from build123d import *

# Parameters (mm, degrees)
SKETCH1_R           = 9.2
BOSS_EXTRUDE1_DEPTH = 65
SKETCH2_W           = 10
SKETCH2_H           = 12.398416249
CUT_EXTRUDE3_DEPTH  = 68.723466712


with BuildPart() as part:
    # Sketch1 → Boss-Extrude1 (new body)
    with BuildSketch(Plane.XY):
        with BuildLine():
            Line((-7, -9.746794345), (-7, -14.746794345))
            Line((-7, -14.746794345), (7, -14.746794345))
            Line((7, -14.746794345), (7, -9.746794345))
            ThreePointArc((7, -9.746794345), (0, 12), (-7, -9.746794345))
        make_face()
        Circle(SKETCH1_R, mode=Mode.SUBTRACT)
    extrude(amount=BOSS_EXTRUDE1_DEPTH)

    # Sketch2 → Cut-Extrude3 (cut, through all)
    with BuildSketch(Plane.XY):
        with Locations((0, -6.800791875)):
            Rectangle(SKETCH2_W, SKETCH2_H)
    extrude(amount=CUT_EXTRUDE3_DEPTH, mode=Mode.SUBTRACT)


solid = part.part
Part model, mm, in its own coordinate system. A direction names the side the tool comes from. Coordinates: 2 decimals unless noted, no trailing zeros. Loops run counter-clockwise (first coordinate to the right, second up) from the corner with the lowest first, then second, coordinate; pieces in that order, holes last. Notation, with made-up numbers: (75.25, 2) -> (89.25, 2) arc R18 cw to (89.25, 23) -> close; hole circle Ø1 at (-40, 11.25). An arc over 180 degrees is marked (long way). Use a Markdown table: item, result. Add a question column.
Item 1: Which spindle directions (+Z, -Z, +X, -X, +Y, -Y) get a long thin tool onto all of the face, cutting with end or side? Do faces 4 (the flat face through (9, 3, 0)), 5 (the flat face through (-7, -12, 32)), 6 (the flat face through (5, -10, 32)). Say none if no direction does.
Item 2: Pull direction X, two halves, no side cores. Call faces 1 (the flat face through (7, -12, 32)), 2 (the flat face through (-5, -10, 32)), 3 (the flat face through (9, 3, 65)): +X half, -X half, draft (parallel to the pull), parting line (faces both ways), or undercut.
Item 3: Flat gauge pins, fed straight in: P1, Ø3, axis at y = 7, z = 55.5, coming from the -X side; P2, Ø1.5, axis at y = -12, z = 47.5, coming from the +X side; P3, Ø3, axis at x = 8.5, z = 47, coming from the +Y side; P4, Ø11, axis at x = 0, y = 0, coming from the -Z side. Where does each tip first touch, or does it go through?
Item 4: Band-saw the part on A-A on y = 0. Write the cut outline in (x, z), plus the area to 3 significant figures.
Item 5: Band-saw the part on B-B on x = 0. Write the cut outline in (y, z), plus the area to 3 significant figures.
Item 6: Probe probe 1 along X at (y, z) = (0, 48.5); probe 2 along Y at (x, z) = (0, 40.5); probe 3 along X at (y, z) = (-10, 54). List the from-to ranges inside material, lowest first.
Item 7: Band-saw the part on C-C on z = 43.5. Write the cut outline in (x, y), plus the area to 3 significant figures.
Geometry says:
| question | item | result |
|---|---|---|
| 1 | face 4 | -Z, +X, -X, +Y, -Y |
| 1 | face 5 | +Z, -Z, -X, -Y |
| 1 | face 6 | +Z, -Z |
| 2 | face 1 | +X half |
| 2 | face 2 | undercut |
| 2 | face 3 | draft |
| 3 | P1 | x = -10.67 |
| 3 | P2 | x = 7 |
| 3 | P3 | y = 9.75 |
| 3 | P4 | through |
| 4 | outline | (-12, 0) -> (-9.2, 0) -> (-9.2, 65) -> (-12, 65) -> close; (9.2, 0) -> (12, 0) -> (12, 65) -> (9.2, 65) -> close |
| 4 | area | 364 mm² |
| 5 | outline | (-14.75, 0) -> (-13, 0) -> (-13, 65) -> (-14.75, 65) -> close; (9.2, 0) -> (12, 0) -> (12, 65) -> (9.2, 65) -> close |
| 5 | area | 296 mm² |
| 6 | probe 1 | -12 to -9.2, 9.2 to 12 |
| 6 | probe 2 | -14.75 to -13, 9.2 to 12 |
| 6 | probe 3 | -7 to -5, 5 to 7 |
| 7 | outline | (-7, -14.75) -> (7, -14.75) -> (7, -9.75) arc R12 ccw (long way) to (-7, -9.75) -> close; hole (-5, -13) -> (5, -13) -> (5, -7.72) arc R9.2 ccw (long way) to (-5, -7.72) -> close |
| 7 | area | 192 mm² |
